Geometry: final body of the model. Coordinates: model frame, mm. Round coordinates to 2 decimals unless told otherwise and drop trailing zeros. Loops run counter-clockwise (first coordinate to the right, second up) from the corner with the lowest first, then second, coordinate; pieces in that order, holes last. Notation, with made-up numbers: M 83,40 L 94,40 A13 cw 94,52 Z; hole C -33,89.5 d5. An arc over 180 degrees is marked long. Return JSON: item names as keys, results as strings.
from build123d import *

# Parameters (mm, degrees)
SKETCH_1_W          = 40
SKETCH_1_H          = 30
EXTRUDE_1_DEPTH     = 3
SKETCH_2_R          = 1.55
CUT_EXTRUDE_1_DEPTH = 26.179356624
SKETCH_3_W          = 40
SKETCH_3_H          = 10
CUT_EXTRUDE_2_DEPTH = 26.179356624
FILLET_2_R          = 3
SKETCH_4_R          = 1.3
CUT_EXTRUDE_3_DEPTH = 26.179356624


with BuildPart() as part:
    # 草图1 → 凸台-拉伸1 (new body)
    with BuildSketch(Plane(origin=(0, 0, 0), x_dir=(1, 0, 0), z_dir=(0, 1, 0))):
        Rectangle(SKETCH_1_W, SKETCH_1_H)
    extrude(amount=EXTRUDE_1_DEPTH)

    # 草图2 → 切除-拉伸1 (cut, through all)
    with BuildSketch(Plane(origin=(0, 3, 0), x_dir=(1, 0, 0), z_dir=(0, 1, 0))):
        with Locations(Location((-10, 0, 0), (0, 0, 270))):
            Circle(SKETCH_2_R)
        with Locations(Location((10, 0, 0), (0, 0, 90))):
            Circle(SKETCH_2_R)
    extrude(amount=-CUT_EXTRUDE_1_DEPTH, mode=Mode.SUBTRACT)

    # 草图3 → 切除-拉伸2 (cut, through all)
    with BuildSketch(Plane(origin=(0, 3, 0), x_dir=(1, 0, 0), z_dir=(0, 1, 0))):
        with Locations((0, 10)):
            Rectangle(SKETCH_3_W, SKETCH_3_H)
    extrude(amount=-CUT_EXTRUDE_2_DEPTH, mode=Mode.SUBTRACT)

    # 圆角2
    fillet_2_edges = [part.edges().sort_by_distance(p)[0] for p in [
        (-20, 1.5, -5),
        (20, 1.5, -5),
        (20, 1.5, 15),
        (-20, 1.5, 15),
    ]]
    fillet(fillet_2_edges, radius=FILLET_2_R)

    # 草图4 → 切除-拉伸3 (cut, through all)
    with BuildSketch(Plane(origin=(0, 3, 0), x_dir=(1, 0, 0), z_dir=(0, 1, 0))):
        with Locations(Location((-12.7, -7, 0), (0, 0, 270))):
            Circle(SKETCH_4_R)
        with Locations(Location((12.7, -7, 0), (0, 0, 90))):
            Circle(SKETCH_4_R)
    extrude(amount=-CUT_EXTRUDE_3_DEPTH, mode=Mode.SUBTRACT)


solid = part.part
Q1. Section query D-D (z = 7). Output: boundary loops of the cut face in (x, y).
Determined:
{"outline": "M -20,0 L -14,0 L -14,3 L -20,3 Z; M -11.4,0 L 11.4,0 L 11.4,3 L -11.4,3 Z; M 14,0 L 20,0 L 20,3 L 14,3 Z"}
Q2. Pin query (flat end, axial travel): pin 1 (2 mm diameter, centred on x = -12.7, z = 7, fed in from +Y). Return the tip coordinate at first contact, or that it passes through.
Determined:
{"pin 1": "passes through"}
Q3. Pull-direction query (X, two-part tool) for faces 1 (the cylindrical face through (12.31, 1.52, 5.76)), 2 (the flat face through (0, 2, -5)), 3 (the cylindrical face through (-11.513, 1.521, -0.336)), 4 (the flat face through (20, 1, 5)); classes: pulls with the +X half, pulls with the -X half, needs draft (parallel to the pull), parting line crosses it, or undercut.
Determined:
{"face 1": "undercut", "face 2": "needs draft", "face 3": "undercut", "face 4": "pulls with the +X half"}
Q4. Section query C-C (y = 0.5). Output: boundary loops of the cut face in (x, z).
Determined:
{"outline": "M -20,-2 A3 ccw -17,-5 L 17,-5 A3 ccw 20,-2 L 20,12 A3 ccw 17,15 L -17,15 A3 ccw -20,12 Z; hole C -12.7,7 d2.6; hole C -10,0 d3.1; hole C 10,0 d3.1; hole C 12.7,7 d2.6"}
Q5. Section query B-B (x = -12.7). Output: boundary loops of the cut face in (y, z), plus the area to 3 significant figures.
Determined:
{"outline": "M 0,-5 L 3,-5 L 3,5.7 L 0,5.7 Z; M 0,8.3 L 3,8.3 L 3,15 L 0,15 Z", "area": "52.2 mm^2"}
Q6. Section query A-A (z = 0). Output: boundary loops of the cut face in (x, y).
Determined:
{"outline": "M -20,0 L -11.55,0 L -11.55,3 L -20,3 Z; M -8.45,0 L 8.45,0 L 8.45,3 L -8.45,3 Z; M 11.55,0 L 20,0 L 20,3 L 11.55,3 Z"}
Q7. Material intervals for L1, parallel to X at y = 1.55, z = 0; L2, parallel to X at y = 2.2, z = 7; L3, parallel to Z at x = 10, y = 1.4, sorted ascending.
Determined:
{"L1": "x = -20 to -11.55, -8.45 to 8.45, 11.55 to 20", "L2": "x = -20 to -14, -11.4 to 11.4, 14 to 20", "L3": "z = -5 to -1.55, 1.55 to 15"}
